Read the model definition and answer for the solid it produces. Units are mm, in the model's axes. Face numbers are marked on the shaded views. A direction names the side the tool comes from. Coordinates: 2 decimals unless noted, no trailing zeros. Write each loop counter-clockwise with the first axis right and the second up, starting at its lowest first coordinate (ties: lowest second). Pieces come first, ordered by that corner, then holes. Notation, with made-up numbers: M 88,35.25 L 147,35.25 A19 ccw 147,68.25 Z; hole C 41.25,64.5 d5. An arc over 180 degrees is marked long. Use a Markdown table: item, result. Add a question column.
from build123d import *

# Parameters (mm, degrees)
F0_W     = 16
F0_H     = 1
F1_DEPTH = 1
F0_W_2   = 20
F2_DEPTH = 10
F3_R     = 0.49999


# Not quite as in the source:
# - a fillet or chamfer is up to 0.001 mm smaller than in the source, because OpenCascade refuses the exact size


with BuildPart() as f1:
    # F0 (on Top) → F1 (new body)
    with BuildSketch(Plane.XY):
        Polygon((10, 1), (-10, 1), (-10, -1), (-8, -1), (8, -1), (10, -1), align=None)
        with Locations((0, -1.5)):
            Rectangle(F0_W, F0_H)
    extrude(amount=F1_DEPTH)

    # F0 (on Top) → F2 (join)
    with BuildSketch(Plane.XY):
        with Locations((0, 1.5)):
            Rectangle(F0_W_2, F0_H)
        Polygon((-8, -1), (-10, -1), (-10, -2), (-9, -2), (-8, -2), align=None)
        Polygon((8, -2), (-8, -2), (-9, -2), (-9, -3), (9, -3), (9, -2), align=None)
        Polygon((10, -2), (10, -1), (8, -1), (8, -2), (9, -2), align=None)
    extrude(amount=F2_DEPTH)

    # F3 (radius 0.5 in the source; OpenCascade refuses exactly that, so slightly less here)
    f3_edges = [f1.edges().sort_by_distance(p)[0] for p in [
        (-9, -2, 5),
        (-9, -3, 5),
        (9, -2, 5),
        (9, -3, 5),
        (-9, -1, 10),
        (-10, -1.5, 10),
        (-9.5, -2, 10),
        (-9, -2.5, 10),
        (0, -3, 10),
        (9, -2.5, 10),
        (9.5, -2, 10),
        (10, -1.5, 10),
        (9, -1, 10),
        (8, -1.5, 10),
        (0, -2, 10),
        (-8, -1.5, 10),
        (-10, 1.5, 10),
        (0, 1, 10),
        (10, 1.5, 10),
        (0, 2, 10),
    ]]
    fillet(f3_edges, radius=F3_R)


solid = f1.part
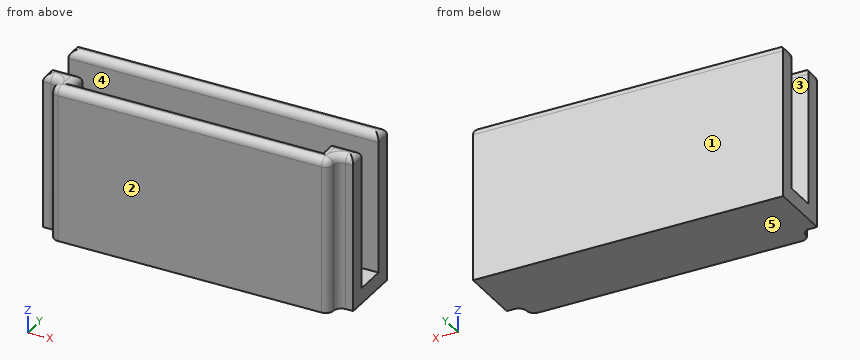
Item 1: Each of these flat-tipped pins is pushed along its axis until it touches: pin 1 (1.5 mm diameter, centred on x = 6, y = 0, fed in from -Z); pin 2 (0.6 mm diameter, centred on x = -9.5, z = 3, fed in from -Y). Where does it stop, or does it pass through?
Item 2: Determine the mould class of the marked faces 1, 2 and 3 for opening direction Y: pulls with the +Y half, pulls with the -Y half, needs draft (parallel to the pull), parting line crosses it, or undercut.
Item 3: Consider probe 1 along X at (y, z) = (-1.85, 9); probe 2 along Y at (x, z) = (2.25, 4.25); probe 3 along Y at (x, z) = (8.5, 6.25). Determine where each line is inside the solid, lowest interval first.
Item 4: For the marked faces 4 and 5, determine the directions among +Z, -Z, +X, -X, +Y, -Y from which every point of the face is accessible in a straight line to the end or side of a thin tool.
Item 5: Find section C-C on y = -0.3. Give the vertices of the cut face in (x, z), then the cut area to 3 significant figures.
Geometry says:
| question | item | result |
|---|---|---|
| 1 | pin 1 | stops at z = 0 |
| 1 | pin 2 | stops at y = -2.1 |
| 2 | face 1 | pulls with the +Y half |
| 2 | face 2 | pulls with the -Y half |
| 2 | face 3 | undercut |
| 3 | probe 1 | x = -10 to -8, 8 to 10 |
| 3 | probe 2 | y = -3 to -2, 1 to 2 |
| 3 | probe 3 | y = -3 to -1, 1 to 2 |
| 4 | face 4 | +Z, +X, -X |
| 4 | face 5 | -Z, +X, -X, +Y, -Y |
| 5 | outline | M -10,0 L 10,0 L 10,1 L -10,1 Z |
| 5 | area | 20.0 mm2 |
